from build123d import *

# Parameters (mm, degrees)
F1_DEPTH      = 14.224
F2_DEPTH      = 7.874
F3_DEPTH      = 12.7
F0_W          = 6.35
F0_H          = 28.575
F4_DEPTH      = 3.048
F4_DEPTH_BACK = 7.874


with BuildPart() as f1:
    # F0 (on Top) → F1 (new body, symmetric)
    with BuildSketch(Plane.XY):
        Polygon((0, 0), (0, 15.875), (-31.492241, 15.875), (-50.951816, 15.875), (-63.246, 15.875), (-69.596, 15.875), (-69.596, 0), (-69.596, -15.875), (-63.246, -15.875), (-50.951816, -15.875), (-31.492241, -15.875), (0, -15.875), align=None)
    extrude(amount=F1_DEPTH, both=True)

    # F0 (on Top) → F2 (join, symmetric)
    with BuildSketch(Plane.XY):
        Polygon((-31.492241, 15.875), (0, 15.875), (6.477, 15.875), (17.526, 26.924), (0, 26.924), (0, 44.45), (-63.246, 44.45), (-63.246, 15.875), (-50.951816, 15.875), align=None)
        with BuildLine():
            ThreePointArc((-50.951816, 24.638), (-56.539816, 30.226), (-50.951816, 35.814))
            Line((-50.951816, 35.814), (-31.565, 36.066451))
            ThreePointArc((-31.565, 36.066451), (-25.904713, 30.551549), (-31.419752, 24.891395))
            Line((-31.419752, 24.891395), (-50.806851, 24.639881))
            ThreePointArc((-50.806851, 24.639881), (-50.879328, 24.63847), (-50.951816, 24.638))
        make_face(mode=Mode.SUBTRACT)
        Polygon((6.477, -15.875), (0, -15.875), (-31.492241, -15.875), (-50.951816, -15.875), (-63.246, -15.875), (-63.246, -44.45), (0, -44.45), (0, -26.924), (17.526, -26.924), align=None)
        with BuildLine():
            Line((-31.565, -36.066451), (-50.951816, -35.814))
            ThreePointArc((-50.951816, -35.814), (-56.539816, -30.226), (-50.951816, -24.638))
            ThreePointArc((-50.951816, -24.638), (-50.879328, -24.63847), (-50.806851, -24.639881))
            Line((-50.806851, -24.639881), (-31.419752, -24.891395))
            ThreePointArc((-31.419752, -24.891395), (-25.904713, -30.551549), (-31.565, -36.066451))
        make_face(mode=Mode.SUBTRACT)
    extrude(amount=F2_DEPTH, both=True)

    # F0 (on Top) → F3 (join, symmetric)
    with BuildSketch(Plane.XY):
        Polygon((0, 26.924), (17.526, 26.924), (35.052, 44.45), (0, 44.45), align=None)
        Polygon((35.052, -44.45), (17.526, -26.924), (0, -26.924), (0, -44.45), align=None)
    extrude(amount=F3_DEPTH, both=True)

    # F0 (on Top) → F4 (join, two sides)
    with BuildSketch(Plane.XY) as f4_sk:
        with Locations((-66.421, 30.1625)):
            Rectangle(F0_W, F0_H)
        with Locations((-66.421, -30.1625)):
            Rectangle(F0_W, F0_H)
    extrude(amount=F4_DEPTH)
    extrude(f4_sk.sketch, amount=-F4_DEPTH_BACK)


solid = f1.part
Geometry: final body of the model. Coordinates: model frame, mm. A direction names the side the tool comes from. Round coordinates to 2 decimals unless told otherwise and drop trailing zeros. Order: outer loops, then holes, each group sorted by start corner. A loop starts at its lowest first (then second) coordinate and runs counter-clockwise, first axis right, second up.
Q1. Pin query (flat end, axial travel): pin 1 (6 mm diameter, centred on x = -5.5, z = 11, fed in from +Y) (3 decimals); pin 2 (1 mm diameter, centred on x = -5, y = -34.5, fed in from +Z); pin 3 (5.5 mm diameter, centred on y = -33, z = 6, fed in from -X). Return the tip coordinate at first contact, or that it passes through.
Result sheet:
pin 1: stops at y = 15.875
pin 2: stops at z = 7.87
pin 3: stops at x = -63.25
Q2. Section D-D, the plane x = 15. Output: boundary loops of the cut face in (y, z).
Result sheet:
outline: (-44.45, -12.7) - (-26.92, -12.7) - (-26.92, -7.87) - (-24.4, -7.87) - (-24.4, 7.87) - (-26.92, 7.87) - (-26.92, 12.7) - (-44.45, 12.7) - close; (24.4, -7.87) - (26.92, -7.87) - (26.92, -12.7) - (44.45, -12.7) - (44.45, 12.7) - (26.92, 12.7) - (26.92, 7.87) - (24.4, 7.87) - close
Q3. Material intervals for probe 1 along Y at (x, z) = (-44, 5.75); probe 2 along Z at (x, y) = (-3.5, -38); probe 3 along Y at (x, z) = (21, 5.25), sorted ascending.
Result sheet:
probe 1: y = -44.45 to -35.9, -24.73 to 24.73, 35.9 to 44.45
probe 2: z = -7.87 to 7.87
probe 3: y = -44.45 to -30.4, 30.4 to 44.45
Q4. Section B-B, the plane x = -20. Output: boundary loops of the cut face in (y, z) (3 decimals), and give its area (3 significant figures).
Result sheet:
outline: (-44.45, -7.874) - (-15.875, -7.874) - (-15.875, -14.224) - (15.875, -14.224) - (15.875, -7.874) - (44.45, -7.874) - (44.45, 7.874) - (15.875, 7.874) - (15.875, 14.224) - (-15.875, 14.224) - (-15.875, 7.874) - (-44.45, 7.874) - close
area: 1,800 mm2
Q5. Mould query, pull axis X, two halves, no side actions, for faces 5 (the face through (0, 36, -10)), 6 (the face through (-34, 15.875, -11)), 7 (the face through (-56.54, 30.1, -0.11)), 8 (the face through (-25.904, -30.429, 0.11)). Classes: released by +X, released by -X, zero draft, split by the parting line, or undercut.
Result sheet:
face 5: released by -X
face 6: zero draft
face 7: undercut
face 8: undercut
Q6. Section C-C, the plane y = 31. Output: boundary loops of the cut face in (x, z).
Result sheet:
outline: (-69.6, -7.87) - (-56.49, -7.87) - (-56.49, 7.87) - (-63.25, 7.87) - (-63.25, 3.05) - (-69.6, 3.05) - close; (-25.93, -7.87) - (0, -7.87) - (0, -12.7) - (21.6, -12.7) - (21.6, 12.7) - (0, 12.7) - (0, 7.87) - (-25.93, 7.87) - close
Q7. Section A-A, the plane z = 11.5. Output: boundary loops of the cut face in (x, y) (3 decimals).
Result sheet:
outline: (-69.596, -15.875) - (0, -15.875) - (0, 15.875) - (-69.596, 15.875) - close; (0, -44.45) - (35.052, -44.45) - (17.526, -26.924) - (0, -26.924) - close; (0, 26.924) - (17.526, 26.924) - (35.052, 44.45) - (0, 44.45) - close
Q8. Access query for faces 1 (the face through (0, 36, 10)), 2 (the face through (24.1, -33.5, 0.2)), 3 (the face through (9, -26.924, -10)), 4 (the face through (0, -36, 10)). Directions: +Z, -Z, +X, -X, +Y, -Y. A direction counts if a zero-diameter tool reaches every point of the face in a straight line with its end or side. Return the directions, or none.
Result sheet:
face 1: +Z, -X, +Y
face 2: +Z, -Z, +X
face 3: -Z, +X, -X
face 4: +Z, -X, -Y
